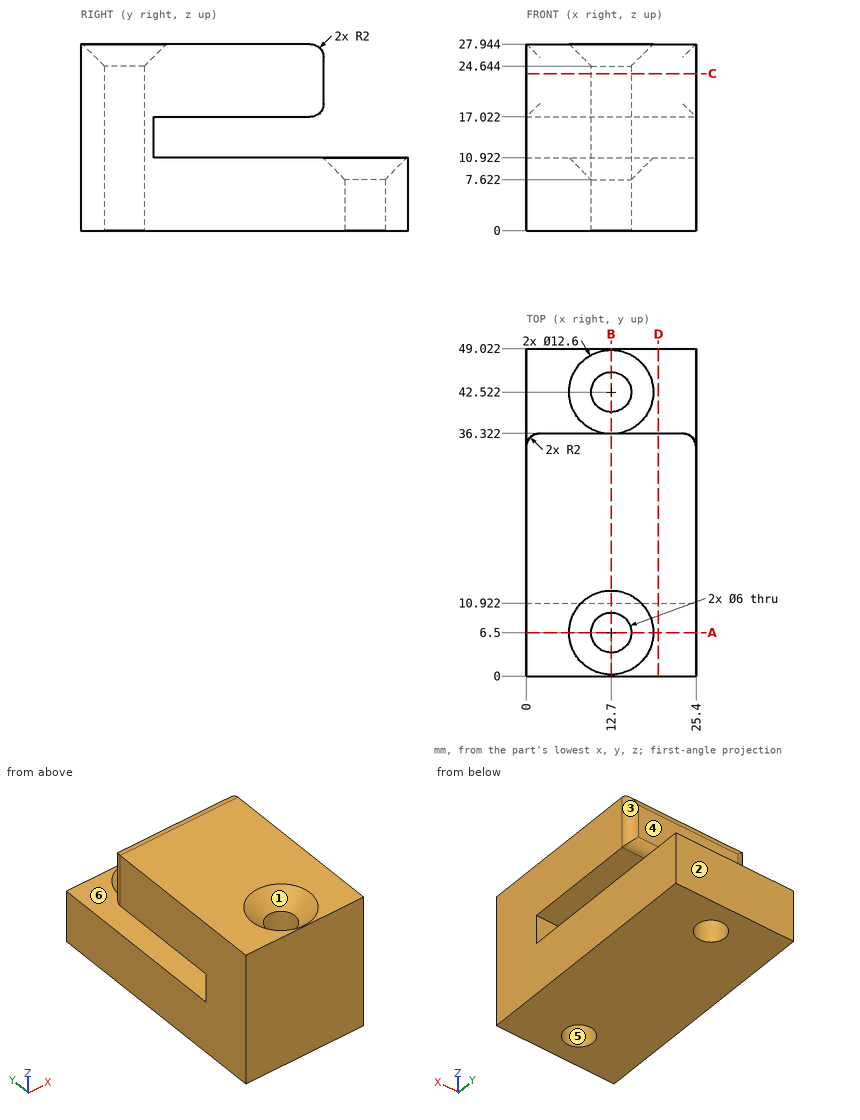
For this review, use the dimensioned drawing (mm, ordinates from the lowest corner) and the shaded views. A direction names the side the tool comes from. Coordinates: 2 decimals unless noted, no trailing zeros. Loops run counter-clockwise (first coordinate to the right, second up) from the corner with the lowest first, then second, coordinate; pieces in that order, holes last.
1. Add section C-C, the plane z = 23.5. Give the boundary of the cut face in (x, y), then the cut area to 3 significant figures.
2. Mouldability with a two-part tool opening along X and no side actions: class the marked faces 1, 2 and 3 as +X half, -X half, draft (parallel to the pull), parting line (faces both ways), or undercut.
3. Add section A-A, the plane y = 6.5. Give the boundary of the cut face in (x, z).
4. Add section D-D, the plane x = 19.75. Give the boundary of the cut face in (y, z).
5. For line 1 (Y direction, x = 12.7, z = 1.5); line 2 (Z direction, x = 24.75, y = 22); line 3 (Y direction, x = 12.7, z = 10), list the stretches that pass through material, from the lowest coordinate up.
6. Add section B-B, the plane x = 12.7. Give the boundary of the cut face in (y, z).
7. For the marked faces 4, 5 and 6, list the 3-axis set-ups (+Z, -Z, +X, -X, +Y, -Y) from which the entire face can be reached by the end or side of a thin tool; tool diameter is ignored.
8. Insertion check: P1, Ø3.5, axis at x = 13.5, z = 22, coming from the +Y side; P2, Ø8, axis at x = 12.7, y = 6.5, coming from the +Z side; P3, Ø9.5, axis at x = 12.7, y = 42.522, coming from the +Z side; P4, Ø2, axis at y = 40, z = 13.5, coming from the +X side. Each pin has a flat end and moves straight along its axis. Give the tip position at first contact, or say it passes through.
Result:
1. outline: (0, 0) - (25.4, 0) - (25.4, 34.32) arc R2 ccw to (23.4, 36.32) - (2, 36.32) arc R2 ccw to (0, 34.32) - close; hole circle Ø6 at (12.7, 6.5)
1. area: 893 mm2
2. face 1: undercut
2. face 2: draft
2. face 3: +X half
3. outline: (0, 0) - (9.7, 0) - (9.7, 24.64) - (6.4, 27.94) - (0, 27.94) - close; (15.7, 0) - (25.4, 0) - (25.4, 27.94) - (19, 27.94) - (15.7, 24.64) - close
4. outline: (0, 0) - (49.02, 0) - (49.02, 10.92) - (10.92, 10.92) - (10.92, 17.02) - (34.32, 17.02) arc R2 ccw to (36.32, 19.02) - (36.32, 25.94) arc R2 ccw to (34.32, 27.94) - (0, 27.94) - close
5. line 1: y = 0 to 3.5, 9.5 to 39.52, 45.52 to 49.02
5. line 2: z = 0 to 10.92, 17.02 to 27.94
5. line 3: y = 0 to 3.5, 9.5 to 37.14, 47.9 to 49.02
6. outline: (0, 0) - (3.5, 0) - (3.5, 24.64) - (0.2, 27.94) - (0, 27.94) - close; (9.5, 0) - (39.52, 0) - (39.52, 7.62) - (36.22, 10.92) - (10.92, 10.92) - (10.92, 17.02) - (34.32, 17.02) arc R2 ccw to (36.32, 19.02) - (36.32, 25.94) arc R2 ccw to (34.32, 27.94) - (12.8, 27.94) - (9.5, 24.64) - close; (45.52, 0) - (49.02, 0) - (49.02, 10.92) - (48.82, 10.92) - (45.52, 7.62) - close
7. face 4: +Z, +X, -X, +Y
7. face 5: +Z, -Z
7. face 6: +X, -X, +Y
8. P1: stops at y = 36.32
8. P2: stops at z = 25.64
8. P3: stops at z = 9.37
8. P4: passes through
